Geometry check sheet. Reference: the model listing, model coordinates, mm. Face numbers are marked on the shaded views. Give positions to 0.01 mm unless a question says otherwise; leave off trailing zeros. Write each loop counter-clockwise with the first axis right and the second up, starting at its lowest first coordinate (ties: lowest second). Pieces come first, ordered by that corner, then holes.
(1) Depth check by flat-ended pin: P1, Ø1.5, axis at x = 1.5, y = -50.5, coming from the -Z side; P2, Ø1, axis at x = 2.5, z = 1, coming from the +Y side; P3, Ø1.5, axis at x = 2.5, y = -59.5, coming from the -Z side; P4, Ø7.5, axis at y = -52.88, z = 0, coming from the +X side. Enter the tip coordinate at first touch or a pass-through.
(2) Cross-section at A-A (z = 0). Record the boundary of the cut face in (x, y).
(3) Thickness scan on line 1 along Z through (x, y) = (6.5, -57); line 2 along Y through (x, z) = (6, -3.25); line 3 along Y through (x, z) = (1, -1.75). Record the ranges inside material, lowest first.
(4) Mould release check, pull along Y, two halves, no side actions. Record for the marked faces 1, 2 and 3: +Y half, -Y half, draft (parallel to the pull), parting line (faces both ways), or undercut.
(5) Cross-section at B-B (x = 5.25). Record the boundary of the cut face in (y, z) (1 decimal), and give its area (3 significant figures).
```python
from build123d import *

# Parameters (mm, degrees)
F0_R     = 11.1125
F0_R_2   = 4.7625
F1_DEPTH = 7.112
F2_SIZE  = 0.508


with BuildPart() as f1:
    # F0 (on Right) → F1 (new body)
    with BuildSketch(Plane.YZ):
        with Locations((-52.88154, 0)):
            Circle(F0_R)
        with Locations((-52.88154, 0)):
            Circle(F0_R_2, mode=Mode.SUBTRACT)
    extrude(amount=F1_DEPTH)

    # F2
    f2_edges = [f1.edges().sort_by_distance(p)[0] for p in [
        (7.112, -63.99404, 0),
        (7.112, -57.64404, 0),
        (0, -63.99404, 0),
        (0, -57.64404, 0),
    ]]
    chamfer(f2_edges, length=F2_SIZE)


solid = f1.part
```
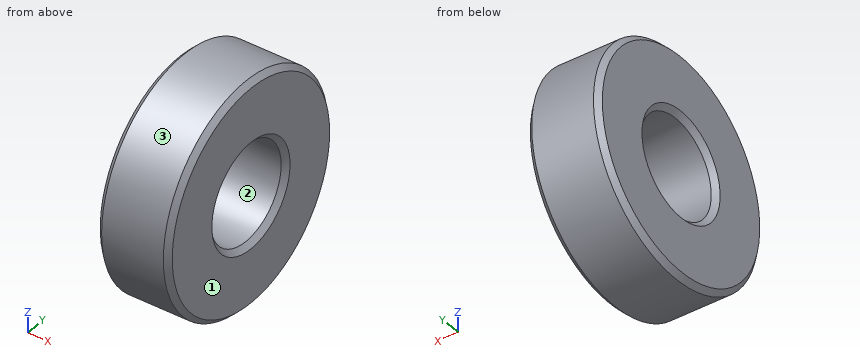
Reply:
1. P1: stops at z = -10.99
1. P2: stops at y = -41.78
1. P3: stops at z = -9.44
1. P4: passes through
2. outline: (0, -63.49) - (0.51, -63.99) - (6.6, -63.99) - (7.11, -63.49) - (7.11, -58.15) - (6.6, -57.64) - (0.51, -57.64) - (0, -58.15) - close; (0, -47.61) - (0.51, -48.12) - (6.6, -48.12) - (7.11, -47.61) - (7.11, -42.28) - (6.6, -41.77) - (0.51, -41.77) - (0, -42.28) - close
3. line 1: z = -10.32 to -2.39, 2.39 to 10.32
3. line 2: y = -63.51 to -56.36, -49.4 to -42.25
3. line 3: y = -63.86 to -57.31, -48.45 to -41.91
4. face 1: draft
4. face 2: undercut
4. face 3: parting line
5. outline: circle Ø22.2 at (-52.9, 0); hole circle Ø9.5 at (-52.9, 0)
5. area: 317 mm2
